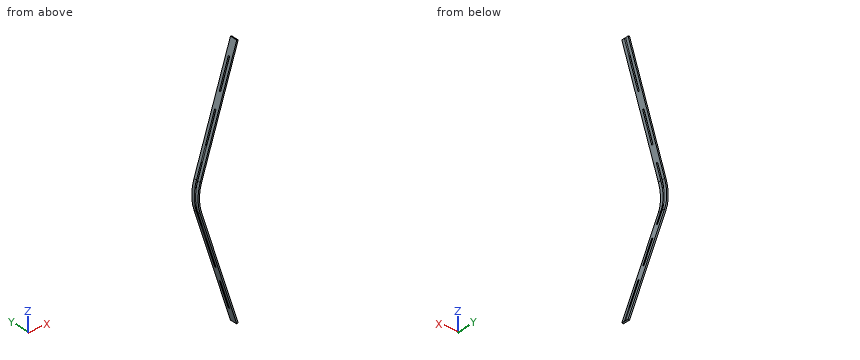
```python
from build123d import *

# Parameters (mm, degrees)
BOSS_EXTRUDE1_DEPTH   = 5
BOSS_EXTRUDE1_2_DEPTH = 5
BOSS_EXTRUDE1_3_DEPTH = 5
BOSS_EXTRUDE1_4_DEPTH = 5
BOSS_EXTRUDE1_5_DEPTH = 5
BOSS_EXTRUDE1_6_DEPTH = 5
BOSS_EXTRUDE1_7_DEPTH = 5
BOSS_EXTRUDE2_DEPTH   = 20
BOSS_EXTRUDE3_DEPTH   = 20


with BuildPart() as part:
    # Sketch3 → Boss-Extrude1 (new body, symmetric)
    with BuildSketch(Plane(origin=(0, 0, 0), x_dir=(1, 0, 0), z_dir=(0, 1, 0))):
        Polygon((-49.523523643, -856.532206403), (-40.006093165, -853.463246139), (-70.69569581, -758.288941363), (-80.213126288, -761.357901628), align=None)
    extrude(amount=BOSS_EXTRUDE1_DEPTH, both=True)



with BuildPart() as body_2:
    # Sketch3 → Boss-Extrude1 2 (new body, symmetric)
    with BuildSketch(Plane(origin=(0, 0, 0), x_dir=(1, 0, 0), z_dir=(0, 1, 0))):
        Polygon((-132.074901101, -567.940331812), (-141.592331578, -571.009292077), (-172.281934223, -475.834987302), (-162.764503746, -472.766027037), align=None)
    extrude(amount=BOSS_EXTRUDE1_2_DEPTH, both=True)


with BuildPart() as body_3:
    # Sketch3 → Boss-Extrude1 3 (new body, symmetric)
    with BuildSketch(Plane(origin=(0, 0, 0), x_dir=(1, 0, 0), z_dir=(0, 1, 0))):
        Polygon((-233.661139514, -285.486377751), (-224.143709036, -282.417417486), (-254.833311681, -187.243112711), (-264.350742159, -190.312072975), align=None)
    extrude(amount=BOSS_EXTRUDE1_3_DEPTH, both=True)


with BuildPart() as body_4:
    # Sketch3 → Boss-Extrude1 4 (new body, symmetric)
    with BuildSketch(Plane(origin=(0, 0, 0), x_dir=(1, 0, 0), z_dir=(0, 1, 0))):
        with BuildLine():
            Line((-305.290403434, -53.830935077), (-295.442325904, -52.0944533))
            ThreePointArc((-295.442325904, -52.0944533), (-300, 0), (-295.442325904, 52.0944533))
            Line((-295.442325904, 52.0944533), (-305.290403434, 53.830935077))
            ThreePointArc((-305.290403434, 53.830935077), (-310, 0), (-305.290403434, -53.830935077))
        make_face()
    extrude(amount=BOSS_EXTRUDE1_4_DEPTH, both=True)


with BuildPart() as body_5:
    # Sketch3 → Boss-Extrude1 5 (new body, symmetric)
    with BuildSketch(Plane(origin=(0, 0, 0), x_dir=(1, 0, 0), z_dir=(0, 1, 0))):
        Polygon((-254.833311681, 187.243112711), (-224.143709036, 282.417417486), (-233.661139514, 285.486377751), (-264.350742159, 190.312072975), align=None)
    extrude(amount=BOSS_EXTRUDE1_5_DEPTH, both=True)


with BuildPart() as body_6:
    # Sketch3 → Boss-Extrude1 6 (new body, symmetric)
    with BuildSketch(Plane(origin=(0, 0, 0), x_dir=(1, 0, 0), z_dir=(0, 1, 0))):
        Polygon((-70.69569581, 758.288941363), (-40.006093165, 853.463246139), (-49.523523643, 856.532206403), (-80.213126288, 761.357901628), align=None)
    extrude(amount=BOSS_EXTRUDE1_6_DEPTH, both=True)


with BuildPart() as body_7:
    # Sketch3 → Boss-Extrude1 7 (new body, symmetric)
    with BuildSketch(Plane(origin=(0, 0, 0), x_dir=(1, 0, 0), z_dir=(0, 1, 0))):
        Polygon((-162.764503746, 472.766027037), (-132.074901101, 567.940331812), (-141.592331578, 571.009292077), (-172.281934223, 475.834987302), align=None)
    extrude(amount=BOSS_EXTRUDE1_7_DEPTH, both=True)


with BuildPart() as part_1:
    add(part.part)

    add(body_2.part)  # Boss-Extrude2 merges body 2

    add(body_3.part)  # Boss-Extrude2 merges body 3

    add(body_4.part)  # Boss-Extrude2 merges body 4

    add(body_5.part)  # Boss-Extrude2 merges body 5

    add(body_6.part)  # Boss-Extrude2 merges body 6

    add(body_7.part)  # Boss-Extrude2 merges body 7
    # Sketch4 → Boss-Extrude2 (add)
    with BuildSketch(Plane(origin=(0, 5, 0), x_dir=(1, 0, 0), z_dir=(0, 1, 0))):
        with BuildLine():
            Line((-49.523523643, 856.532206403), (-40.006093165, 853.463246139))
            Line((-40.006093165, 853.463246139), (-285.522914326, 92.068807935))
            ThreePointArc((-285.522914326, 92.068807935), (-300, 0), (-285.522914326, -92.068807935))
            Line((-285.522914326, -92.068807935), (-40.006093165, -853.463246139))
            Line((-40.006093165, -853.463246139), (-49.523523643, -856.532206403))
            Line((-49.523523643, -856.532206403), (-295.040344804, -95.1377682))
            ThreePointArc((-295.040344804, -95.1377682), (-310, 0), (-295.040344804, 95.1377682))
            Line((-295.040344804, 95.1377682), (-49.523523643, 856.532206403))
        make_face()
    extrude(amount=BOSS_EXTRUDE2_DEPTH)

    # Sketch5 → Boss-Extrude3 (add)
    with BuildSketch(Plane.XZ.offset(5)):
        with BuildLine():
            Line((-49.523523643, 856.532206403), (-40.006093165, 853.463246139))
            Line((-40.006093165, 853.463246139), (-285.522914326, 92.068807935))
            ThreePointArc((-285.522914326, 92.068807935), (-300, 0), (-285.522914326, -92.068807935))
            Line((-285.522914326, -92.068807935), (-40.006093165, -853.463246139))
            Line((-40.006093165, -853.463246139), (-49.523523643, -856.532206403))
            Line((-49.523523643, -856.532206403), (-295.040344804, -95.1377682))
            ThreePointArc((-295.040344804, -95.1377682), (-310, 0), (-295.040344804, 95.1377682))
            Line((-295.040344804, 95.1377682), (-49.523523643, 856.532206403))
        make_face()
    extrude(amount=BOSS_EXTRUDE3_DEPTH)


solid = part_1.part
```
Geometry check sheet. Reference: the model listing, model coordinates, mm. Give positions to 0.01 mm unless a question says otherwise; leave off trailing zeros. Loops run counter-clockwise (first coordinate to the right, second up) from the corner with the lowest first, then second, coordinate; pieces in that order, holes last. Notation, with made-up numbers: M -13,-31 L -4,-31 A21 ccw -4,-14 Z; hole C -1,-34 d4. An arc over 180 degrees is marked long. Write item = value, one per line. Start each with the question number.
1. Thickness scan on probe 1 along X at (y, z) = (12, 526.5); probe 2 along X at (y, z) = (8, -102). Record the ranges inside material, lowest first.
2. Section check B-B, the plane y = 12.5. Enter the section's corners in (x, z).
3. Section check C-C, the plane z = 212.5. Enter the section's corners in (x, y).
4. Section check A-A, the plane z = -454.5. Enter the section's corners in (x, y).
5. Go/stop test with flat-tipped pins: P1, Ø2, axis at y = 18.5, z = -398.5, coming from the -X side; P2, Ø21.5, axis at x = -97.5, z = 624, coming from the +Y side; P3, Ø8, axis at y = 11, z = -529, coming from the +X side; P4, Ø4, axis at y = -12, z = -128.5, coming from the +X side. Record where each tip stops, or that it passes through.
Values follow:
q1.probe_1 = -155.94 to -145.44
q1.probe_2 = -292.83 to -282.32
q2.outline = M -295.04,-95.14 L -49.52,-856.53 L -40.01,-853.46 L -285.52,-92.07 A300 cw -285.52,92.07 L -40.01,853.46 L -49.52,856.53 L -295.04,95.14 A310 ccw Z
q3.outline = M -257.2,-25 L -246.69,-25 L -246.69,25 L -257.2,25 Z
q4.outline = M -179.16,-25 L -168.65,-25 L -168.65,-5 L -179.16,-5 Z; M -179.16,5 L -168.65,5 L -168.65,25 L -179.16,25 Z
q5.P1 = -197.54
q5.P2 = through
q5.P3 = -143.34
q5.P4 = -273.13
